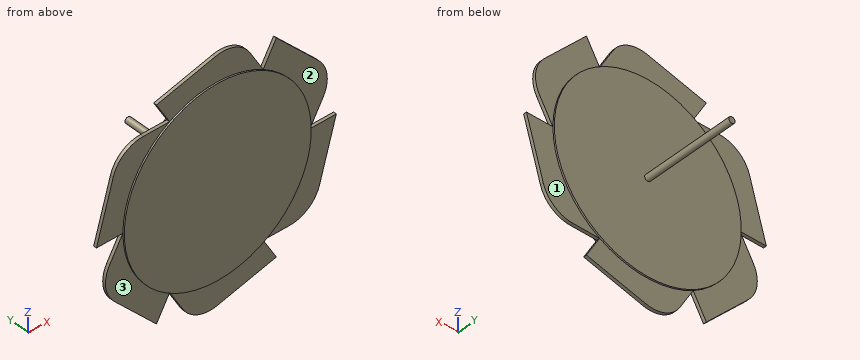
from build123d import *

# Parameters (mm, degrees)
SKETCH1_R           = 15
BOSS_EXTRUDE1_DEPTH = 0.5
BOSS_EXTRUDE3_DEPTH = 0.25
SKETCH2_R           = 0.5
BOSS_EXTRUDE4_DEPTH = 15


with BuildPart() as part:
    # Sketch1 → Boss-Extrude1 (new, symmetric)
    with BuildSketch(Plane(origin=(0, 0, 0), x_dir=(1, 0, 0), z_dir=(0, 1, 0))):
        with Locations(Location((0, 0, 0), (0, 0, 270))):
            Circle(SKETCH1_R)
    extrude(amount=BOSS_EXTRUDE1_DEPTH, both=True)

    # Sketch1_3 → Boss-Extrude3 (add, symmetric)
    with BuildSketch(Plane(origin=(0, 0, 0), x_dir=(1, 0, 0), z_dir=(0, 1, 0))):
        with BuildLine():
            ThreePointArc((-7.5, -12.990381057), (-12.990381057, -7.5), (-15, 0))
            Line((-15, 0), (-19.2350492, 0))
            Line((-19.2350492, 0), (-16.540364811, -9.372025687))
            ThreePointArc((-16.540364811, -9.372025687), (-14.742687547, -11.984640885), (-11.7350492, -12.990381057))
            Line((-11.7350492, -12.990381057), (-7.5, -12.990381057))
        make_face()
        with BuildLine():
            ThreePointArc((-15, 0), (-12.990381057, 7.5), (-7.5, 12.990381057))
            Line((-7.5, 12.990381057), (-9.6175246, 16.658041251))
            Line((-9.6175246, 16.658041251), (-16.386594735, 9.638363271))
            ThreePointArc((-16.386594735, 9.638363271), (-17.750347235, 6.775221493), (-17.1175246, 3.667660194))
            Line((-17.1175246, 3.667660194), (-15, 0))
        make_face()
        with BuildLine():
            Line((-5.3824754, 16.658041251), (-7.5, 12.990381057))
            ThreePointArc((-7.5, 12.990381057), (0, 15), (7.5, 12.990381057))
            Line((7.5, 12.990381057), (9.6175246, 16.658041251))
            Line((9.6175246, 16.658041251), (0.153770076, 19.010388957))
            ThreePointArc((0.153770076, 19.010388957), (-3.007659688, 18.759862378), (-5.3824754, 16.658041251))
        make_face()
        with BuildLine():
            Line((11.7350492, 12.990381057), (7.5, 12.990381057))
            ThreePointArc((7.5, 12.990381057), (12.990381057, 7.5), (15, 0))
            Line((15, 0), (19.2350492, 0))
            Line((19.2350492, 0), (16.540364811, 9.372025687))
            ThreePointArc((16.540364811, 9.372025687), (14.742687547, 11.984640885), (11.7350492, 12.990381057))
        make_face()
        with BuildLine():
            Line((17.1175246, -3.667660194), (15, 0))
            ThreePointArc((15, 0), (12.990381057, -7.5), (7.5, -12.990381057))
            Line((7.5, -12.990381057), (9.6175246, -16.658041251))
            Line((9.6175246, -16.658041251), (16.386594735, -9.638363271))
            ThreePointArc((16.386594735, -9.638363271), (17.750347235, -6.775221493), (17.1175246, -3.667660194))
        make_face()
        with BuildLine():
            ThreePointArc((7.5, -12.990381057), (0, -15), (-7.5, -12.990381057))
            Line((-7.5, -12.990381057), (-9.6175246, -16.658041251))
            Line((-9.6175246, -16.658041251), (-0.153770076, -19.010388957))
            ThreePointArc((-0.153770076, -19.010388957), (3.007659688, -18.759862378), (5.3824754, -16.658041251))
            Line((5.3824754, -16.658041251), (7.5, -12.990381057))
        make_face()
    extrude(amount=BOSS_EXTRUDE3_DEPTH, both=True)

    # Sketch2 → Boss-Extrude4 (add)
    with BuildSketch(Plane(origin=(0, 0.5, 0), x_dir=(1, 0, 0), z_dir=(0, 1, 0))):
        with Locations(Location((0, 0, 0), (0, 0, 270))):
            Circle(SKETCH2_R)
    extrude(amount=BOSS_EXTRUDE4_DEPTH)


solid = part.part
Model file for the job. Use its own axes, mm. Face numbers are marked on the shaded views. A direction names the side the tool comes from. Give positions to 0.01 mm unless a question says otherwise; leave off trailing zeros. Loops run counter-clockwise (first coordinate to the right, second up) from the corner with the lowest first, then second, coordinate; pieces in that order, holes last.
Item 1: Drill centre lines: line 1 along Y through (x, z) = (-6, -3.5); line 2 along Y through (x, z) = (-11, -11). Where is each one in solid material? Low to high.
Check values:
line 1: y = -0.5 to 0.5
line 2: y = -0.25 to 0.25
Item 2: Slice it at D-D (x = 15.5). Write the cut outline in (y, z), plus the area to 3 significant figures.
Check values:
outline: (-0.25, -11.28) - (0.25, -11.28) - (0.25, 0) - (-0.25, 0) - close; (-0.25, 0.87) - (0.25, 0.87) - (0.25, 10.56) - (-0.25, 10.56) - close
area: 10.5 mm2
Item 3: Drop flat-ended pins along their axis: P1, Ø5, axis at x = -15, z = 8, coming from the -Y side; P2, Ø13, axis at x = 13, z = -9, coming from the +Y side; P3, Ø3, axis at x = 3, z = -16.5, coming from the +Y side; P4, Ø8, axis at x = -11, y = 2, coming from the +Z side. Give the stop position or say it passes through.
Check values:
P1: stops at y = -0.5
P2: stops at y = 0.5
P3: stops at y = 0.25
P4: stops at z = 17.21
Item 4: Slice it at C-C (y = 13). Write the cut outline in (x, z).
Check values:
outline: circle Ø1 at (0, 0)
Item 5: Slice it at B-B (z = -8.5). Write the cut outline in (x, y), plus the area to 3 significant figures.
Check values:
outline: (-17.21, -0.25) - (-12.36, -0.25) - (-12.36, -0.5) - (12.36, -0.5) - (12.36, -0.25) - (16.79, -0.25) - (16.79, 0.25) - (12.36, 0.25) - (12.36, 0.5) - (-12.36, 0.5) - (-12.36, 0.25) - (-17.21, 0.25) - close
area: 29.4 mm2
Item 6: Slice it at A-A (x = 8). Write the cut outline in (y, z), plus the area to 3 significant figures.
Check values:
outline: (-0.5, -12.69) - (-0.25, -12.69) - (-0.25, -12.99) - (0.25, -12.99) - (0.25, -12.69) - (0.5, -12.69) - (0.5, 12.69) - (0.25, 12.69) - (0.25, 13.86) - (-0.25, 13.86) - (-0.25, 12.69) - (-0.5, 12.69) - close; (-0.25, -17.06) - (0.25, -17.06) - (0.25, -13.86) - (-0.25, -13.86) - close
area: 27.7 mm2
Item 7: Which spindle directions (+Z, -Z, +X, -X, +Y, -Y) get a long thin tool onto all of the face, cutting with end or side? Do the marked faces 1, 2 and 3. Say none if no direction does.
Check values:
face 1: -Z, +X, +Y
face 2: +Z, +X, -Y
face 3: -Z, -X, -Y
